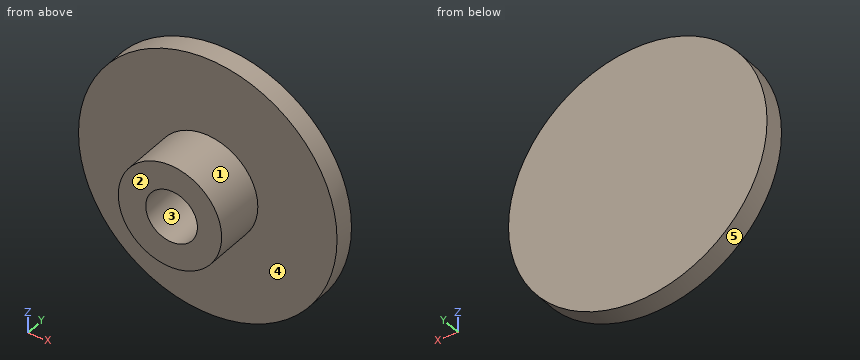
Autodesk Inventor part; units mm, degrees
ref_plane "YZ Plane" through (0, 0, 0) normal (1, 0, 0) x (0, 1, 0)
ref_plane "XZ Plane" through (0, 0, 0) normal (0, 1, 0) x (-1, 0, 0)
ref_plane "XY Plane" through (0, 0, 0) normal (0, 0, 1) x (1, 0, 0)
sketch "Sketch1" plane through (0, 0, 0) normal (0, 1, 0) x (-1, 0, 0)
  circle A0 centre (0, 0) radius 12.5
  dimension "d0" = 25
extrude "Extrusion1" add sketch "Sketch1" along normal blind 2
sketch "Sketch2" plane through (0, 0, 0) normal (0, -1, 0) x (1, 0, 0)
  circle A0 centre (0, 0) radius 2.5
  circle A1 centre (-0.1585, 0) radius 5
  dimension "d3" = 5
  dimension "d4" = 10
extrude "Extrusion2" add sketch "Sketch2" along normal blind 5
equation "\"BendRadius\" = Thickness"
equation "\"BendReliefWidth\" = Thickness"
equation "\"BendReliefDepth\" = 0.5 * Thickness"
equation "\"CornerReliefSize\" = 4 * Thickness"
equation "\"MinimumRemnant\" = 2 * Thickness"
equation "\"TransitionRadius\" = BendRadius"
equation "\"JacobiRadiusSize\" = BendRadius"
equation "\"GapSize\" = Thickness"
properties part number "Servo_bigg_top"
The listing builds one solid part. Answer for the finished solid, in the listing's coordinates (mm). Face numbers are marked on the shaded views. A direction names the side the tool comes from. Coordinates: 2 decimals unless noted, no trailing zeros. Write each loop counter-clockwise with the first axis right and the second up, starting at its lowest first coordinate (ties: lowest second). Pieces come first, ordered by that corner, then holes. Notation, with made-up numbers: (49.25, 14) - (94.25, 14) arc R30 cw to (94.25, 40) - close; hole circle Ø4 at (29.25, -30). An arc over 180 degrees is marked (long way). Return JSON: item names as keys, results as strings. Group by question number.
1. A cutting plane is placed at B-B, the plane x = 0. Determine the outline of the cut face in (y, z).
2. Which of the six approach directions +Z, -Z, +X, -X, +Y, -Y give full straight-line access (tool end or side, diameter ignored) to the marked faces 4 and 5?
3. Straight lines are drawn through the part: L1, parallel to Z at x = 0, y = -2.4; L2, parallel to Y at x = -6.5, z = 10.25; L3, parallel to Z at x = -5, y = 0.5. For each, find the intervals that lie inside material, in ascending order.
4. A cutting plane is placed at A-A, the plane z = 0. Determine the outline of the cut face in (x, y), plus the area to 3 significant figures.
5. A cutting plane is placed at C-C, the plane y = 1.5. Determine the outline of the cut face in (x, z), plus the area to 3 significant figures.
6. A cutting plane is placed at D-D, the plane y = -1.25. Determine the outline of the cut face in (x, z).
7. Determine the mould class of the marked faces 1, 2 and 3 for opening direction X: released by +X, released by -X, zero draft, split by the parting line, or undercut.
8. Given pin 1 (1 mm diameter, centred on y = 0, z = -1.5, fed in from +X); pin 2 (1 mm diameter, centred on x = -2, y = -3, fed in from -Z); pin 3 (1 mm diameter, centred on x = 4, y = -4, fed in from -Z), each flat-ended and moving along its own axis, determine where each tip first touches the part or whether it passes through.
Ans:
{
 "1": {"outline": "(-5, -5) - (0, -5) - (0, -12.5) - (2, -12.5) - (2, 12.5) - (0, 12.5) - (0, 5) - (-5, 5) - (-5, 2.5) - (0, 2.5) - (0, -2.5) - (-5, -2.5) - close"},
 "2": {"face 4": "-Y", "face 5": "+Y, -Y"},
 "3": {"L1": "-5 to -2.5, 2.5 to 5", "L2": "0 to 2", "L3": "-11.46 to 11.46"},
 "4": {"outline": "(-12.5, 0) - (-5.16, 0) - (-5.16, -5) - (-2.5, -5) - (-2.5, 0) - (2.5, 0) - (2.5, -5) - (4.84, -5) - (4.84, 0) - (12.5, 0) - (12.5, 2) - (-12.5, 2) - close", "area": "75.0 mm²"},
 "5": {"outline": "circle Ø25 at (0, 0)", "area": "491 mm²"},
 "6": {"outline": "circle Ø10 at (-0.16, 0); hole circle Ø5 at (0, 0)"},
 "7": {"face 1": "split by the parting line", "face 2": "zero draft", "face 3": "undercut"},
 "8": {"pin 1": "x = 12.46", "pin 2": "z = -4.82", "pin 3": "z = -3.41"}
}
